Here's the drawing with two shaded views (mm, measured from the low corner). I have some questions. A direction names the side the tool comes from. Coordinates: 2 decimals unless noted, no trailing zeros. Write each loop counter-clockwise with the first axis right and the second up, starting at its lowest first coordinate (ties: lowest second). Pieces come first, ordered by that corner, then holes. Notation, with made-up numbers: (64.25, 47) -> (74.25, 47) arc R20 ccw to (74.25, 81) -> close; hole circle Ø10 at (-27.5, 63). An arc over 180 degrees is marked (long way). Use a Markdown table: item, result. Add a question column.
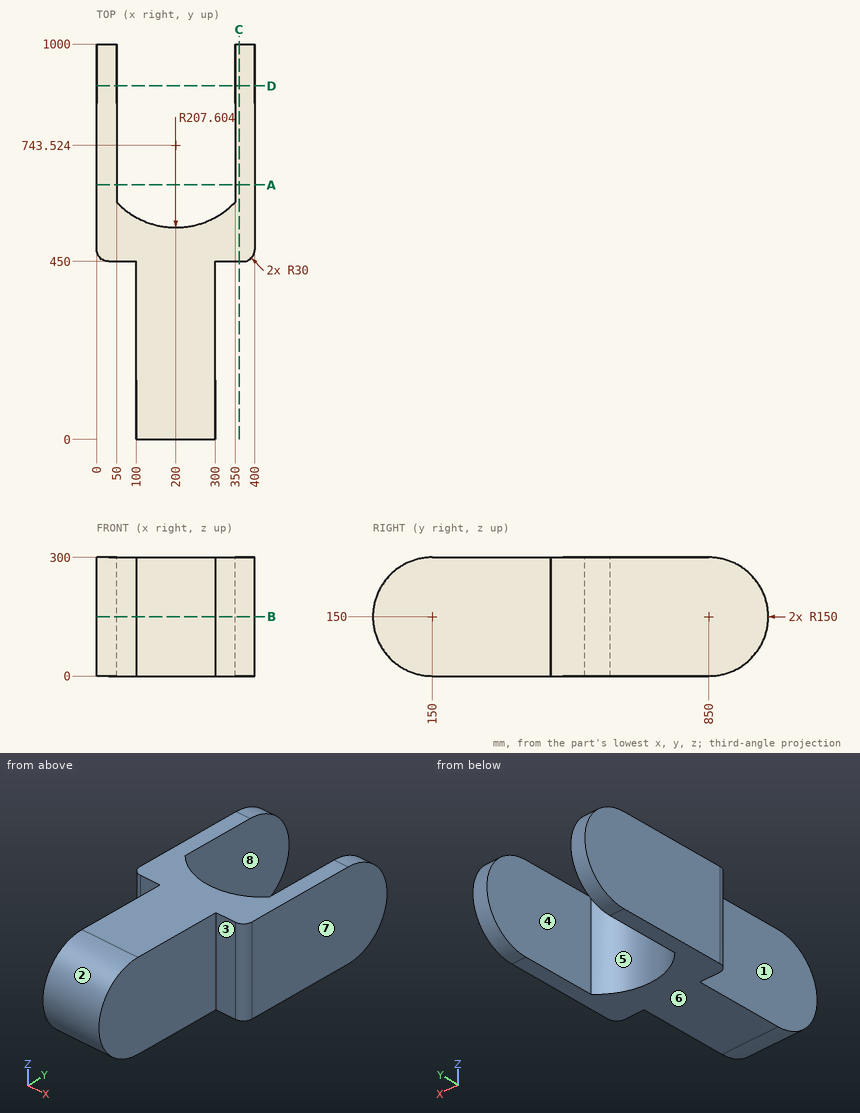
Q1. Suppose I cut it at D-D, the plane y = 894. Write out the boundary of the cut face in (x, z), and give its area (3 significant figures).
Q2. Which directions (+Z, -Z, +X, -X, +Y, -Y) give clear straight access to the entire face, cutting with the end or side of a thin tool? Please do the marked faces 1, 2, 3 and 4.
Q3. Suppose I cut it at C-C, the plane x = 360. Write out the boundary of the cut face in (y, z).
Q4. Suppose I cut it at A-A, the plane y = 644. Write out the boundary of the cut face in (x, z), and give its area (3 significant figures).
Q5. Please list where these lines run through material, in increasing order: line 1 (X direction, y = 637, z = 171.5); line 2 (X direction, y = 443, z = 87.5); line 3 (Y direction, x = 23, z = 138.5).
Q6. Will these pins go through, and if not, where does the flat tip stop? pin 1 (6 mm diameter, centred on x = 75, z = 58, fed in from +Y) (1 decimal); pin 2 (21 mm diameter, centred on x = 75, z = 88, fed in from -Y); pin 3 (5 mm diameter, centred on x = 128.5, z = 33.5, fed in from -Y).
Q7. Thinking about a two-plate mould opening in X: for the marked faces 5, 6, 7 and 8, which applies, released by +X, released by -X, zero draft, split by the parting line, or undercut?
Q8. Suppose I cut it at B-B, the plane z = 150. Write out the boundary of the cut face in (x, y) (1 decimal).
Answer key:
| question | item | result |
|---|---|---|
| 1 | outline | (0, 6.6) -> (50, 6.6) -> (50, 293.4) -> (0, 293.4) -> close; (350, 6.6) -> (400, 6.6) -> (400, 293.4) -> (350, 293.4) -> close |
| 1 | area | 28,700 mm^2 |
| 2 | face 1 | +Z, -Z, -X, -Y |
| 2 | face 2 | +X, -X, -Y |
| 2 | face 3 | +Z, -Z, +X, -Y |
| 2 | face 4 | +Z, -Z, +Y |
| 3 | outline | (450, 0) -> (850, 0) arc R150 ccw to (850, 300) -> (450, 300) -> close |
| 4 | outline | (0, 0) -> (50, 0) -> (50, 300) -> (0, 300) -> close; (350, 0) -> (400, 0) -> (400, 300) -> (350, 300) -> close |
| 4 | area | 30,000 mm^2 |
| 5 | line 1 | x = 0 to 50, 350 to 400 |
| 5 | line 2 | x = 100 to 300 |
| 5 | line 3 | y = 450.83 to 999.56 |
| 6 | pin 1 | stops at y = 580.1 |
| 6 | pin 2 | stops at y = 450 |
| 6 | pin 3 | stops at y = 52.51 |
| 7 | face 5 | undercut |
| 7 | face 6 | zero draft |
| 7 | face 7 | released by +X |
| 7 | face 8 | undercut |
| 8 | outline | (0, 480) arc R30 ccw to (30, 450) -> (100, 450) -> (100, 0) -> (300, 0) -> (300, 450) -> (370, 450) arc R30 ccw to (400, 480) -> (400, 1000) -> (350, 1000) -> (350, 600) arc R207.6 cw to (50, 600) -> (50, 1000) -> (0, 1000) -> close |
